Build history of the part. All positions in model axes, mm. A direction names the side the tool comes from. Give positions to 0.01 mm unless a question says otherwise; leave off trailing zeros. Write each loop counter-clockwise with the first axis right and the second up, starting at its lowest first coordinate (ties: lowest second). Pieces come first, ordered by that corner, then holes. Notation, with made-up numbers: M 63.5,59 L 81.5,59 A30 cw 81.5,86 Z; hole C -18.5,-7 d4. An arc over 180 degrees is marked long. One line per item, written item: value. Start each with the question number.
Autodesk Inventor part; units mm, degrees
ref_plane "YZ Plane" through (0, 0, 0) normal (1, 0, 0) x (0, 1, 0)
ref_plane "XZ Plane" through (0, 0, 0) normal (0, 1, 0) x (-1, 0, 0)
ref_plane "XY Plane" through (0, 0, 0) normal (0, 0, 1) x (1, 0, 0)
sketch "Sketch1" plane through (0, 0, 0) normal (0, 1, 0) x (-1, 0, 0)
  line L0 (0, 0) -> (12, 0) construction
  line L1 (12, 24) -> (12, -24) construction
  circle A0 centre (12, 24) radius 1.5
  circle A1 centre (12, -24) radius 1.5
  line L2 (15, 27.5) -> (15, 20.5)
  line L3 (15, 20.5) -> (4, 20.5)
  line L4 (4, 20.5) -> (4, 0)
  line L5 (15, 27.5) -> (-16, 27.5)
  line L6 (4, 0) -> (12, 0) construction
  line L7 (15, -27.5) -> (15, -20.5)
  line L8 (15, -20.5) -> (4, -20.5)
  line L9 (4, -20.5) -> (4, 0)
  line L10 (15, -27.5) -> (-16, -27.5)
  line L11 (12, 24) -> (15, 24) construction
  line L12 (-16, 27.5) -> (-16, -27.5)
  line L13 (0, 27.5) -> (0, -27.5)
  line L14 (4, 20.5) -> (4, 27.5)
  line L15 (4, -20.5) -> (4, -27.5)
  circle A2 centre (-3, 8) radius 1
  circle A3 centre (-3, 19.5) radius 1
  line L16 (-3, 8) -> (-3, 19.5) construction
  circle A4 centre (-5, -24.5) radius 1
  circle A5 centre (-5, -6) radius 1
  line L17 (-5, -24.5) -> (-5, -6) construction
  arc A6 (-16, -27.5) -> (-11, -27.5) centre (-13.5, -27.5) ccw
  arc A7 (-15, -27.5) -> (-12, -27.5) centre (-13.5, -27.5) ccw
  point P0 (-12, -27.5)
  dimension "d0" = 3
  dimension "d1" = 3
  dimension "d2" = 3
  dimension "d3" = 7
  dimension "d4" = 48
  dimension "d5" = 8
  dimension "d7" = 4
  dimension "d12" = 20
  dimension "d13" = 2
  dimension "d14" = 2
  dimension "d15" = 11.5
  dimension "d16" = 3
  dimension "d17" = 2
  dimension "d18" = 2
  dimension "d19" = 18.5
  dimension "d20" = 5
  dimension "d23" = 8
  dimension "d24" = 3
  dimension "d27" = 5
  dimension "d28" = 1
extrude "Extrusion1" add sketch "Sketch1" along normal blind 2 contours L2 L3 L14 L5 | L14 L4 L9 L15 L10 L13 L5 | L8 L7 L10 L15
extrude "Extrusion2" add sketch "Sketch1" against normal blind 14 contours L14 L4 L9 L15 L10 L13 L5
extrude "Extrusion3" add sketch "Sketch1" along normal blind 2 from surface at -14 contours L13 L10 L12 L5 | L10 A7 A6
sketch "Sketch2" plane through (0, 2, 27.5) normal (1, 0, 0) x (0, 0, -1)
  line L0 (55, -14) -> (0, -14)
  line L1 (55, -14) -> (55, 0)
  line L2 (0, 0) -> (55, 0)
  line L3 (0, -14) -> (0, 0)
  line L4 (32.5, -14) -> (34.5, -14)
  line L5 (51, -14) -> (53, -14)
  line L6 (33.5, -14) -> (52, -14)
  line L7 (42.75, -14) -> (42.75, -6) construction
  line L8 (42.75, -6) -> (37.75, -6)
  line L9 (37.75, -6) -> (37.75, -14)
  line L10 (42.75, -6) -> (47.75, -6)
  line L11 (47.75, -6) -> (47.75, -14)
  point P0 (27.5, -2)
  dimension "d29" = 10
  dimension "d30" = 8
extrude "Extrusion4" cut sketch "Sketch2" against normal through all contours L0 L9 L8 L10 L11
chamfer "Chamfer1" distance 5 distance2 4 2 edges at (-2, -4, -10.25) (-2, -4, -20.25) measured on face at (-2.6667, -4, -13.5833)
equation "\"d14\" = d13"
equation "\"d18\" = d17"
properties part number "adcDAcmount_3DPrint"
1) Probe line 1 along Z through (x, y) = (-12, 0.6); line 2 along Z through (x, y) = (5, -12.95); line 3 along Z through (x, y) = (3, -13.2). List the from-to ranges inside material, lowest first. Write a range as from..to.
2) Band-saw the part on B-B (y = 1.25). List the corners of the cut face in (x, z).
3) Band-saw the part on A-A (z = 24). List the corners of the cut face in (x, y), then the cut area to 3 significant figures.
4) Tool access for faces 1 (the face through (13.4, -13, -30)), 2 (the face through (-2, -5, -27.5)), 3 (the face through (-1.97, -6.03, -17.79)): list every direction of +Z, -Z, +X, -X, +Y, -Y with a clear straight run to the whole face (end or side of a thin tool).
5) Drop flat-ended pins along their axis: P1, Ø5, axis at x = 1.5, z = 18, coming from the +Y side; P2, Ø2.5, axis at x = -12, z = -24, coming from the -Y side; P3, Ø5.5, axis at x = -8.5, z = -24.5, coming from the -Y side; P4, Ø4, axis at x = -1.5, y = -9, coming from the -Z side. Give the stop position or say it passes through.
6) Band-saw the part on D-D (y = -9). List the corners of the cut face in (x, z), then the cut area to 3 significant figures.
7) Band-saw the part on C-C (x = -6.5). List the corners of the cut face in (y, z), then the cut area to 3 significant figures.
8) Mould opens along Y. For faces 4 (the face through (-2, -10, -10.25)), 5 (the face through (-1.97, -6.03, -12.71)), 6 (the face through (-9, 0, 24)), 7 (the face through (5, -13, -7)) say: released by +Y, released by -Y, zero draft, split by the parting line, or undercut.
Model answer:
1. line 1: z = -27.5..-25.5, -22.5..-20.5, 20.5..22.5, 25.5..27.5
1. line 2: z = -27.5..-25.5, -23.5..-7, -5..27.5
1. line 3: z = -27.5..7, 9..18.5, 20.5..27.5
2. outline: M -15,-27.5 L 0,-27.5 L 0,27.5 L -15,27.5 L -15,20.5 L -4,20.5 L -4,-20.5 L -15,-20.5 Z; hole C -12,-24 d3; hole C -12,24 d3
3. outline: M -15,0 L -13.5,0 L -13.5,2 L -15,2 Z; M -10.5,0 L -4,0 L -4,-14 L 16,-14 L 16,-12 L 0,-12 L 0,2 L -10.5,2 Z
3. area: 112 mm²
4. face 1: -Z, +Y, -Y
4. face 2: -Z, -X, +Y, -Y
4. face 3: +X, -X
5. P1: stops at y = 2
5. P2: passes through
5. P3: stops at y = 0
5. P4: stops at z = -27.5
6. outline: M -4,-27.5 L 0,-27.5 L 0,-20.25 L -4,-20.25 Z; M -4,-10.25 L 0,-10.25 L 0,27.5 L -4,27.5 Z
6. area: 180 mm²
7. outline: M 0,-27.5 L 2,-27.5 L 2,-20.5 L 0,-20.5 Z; M 0,20.5 L 2,20.5 L 2,27.5 L 0,27.5 Z
7. area: 28.0 mm²
8. face 4: undercut
8. face 5: undercut
8. face 6: released by -Y
8. face 7: zero draft
